Solid Edge part; units mm, degrees
sketch "Sketch1" plane through (0, 0, 0) normal (0, 0, 1) x (1, 0, 0)
  line L0 (-28, -63) -> (28, -63)
  line L1 (28, -63) -> (28, 24)
  line L2 (28, 24) -> (-28, 24)
  line L3 (-28, 24) -> (-28, -63)
  circle A0 centre (-23, -43) radius 1.7
  circle A1 centre (23, -43) radius 1.7
  circle A2 centre (-23, 18) radius 1.7
  circle A3 centre (23, 18) radius 1.7
extrude "Protrusion1" add sketch "Sketch1" along normal blind 6
sketch "Sketch2" plane through (0, 0, 6) normal (0, 0, 1) x (1, 0, 0)
  line L0 (-28, -63) -> (28, -63)
  line L1 (28, -63) -> (28, -55)
  line L2 (28, -55) -> (-28, -55)
  line L3 (-28, -55) -> (-28, -63)
extrude "ExtrudedProtrusion_2" add sketch "Sketch2" along normal blind 24
sketch "Sketch3" plane through (0, 0, 6) normal (0, 0, 1) x (1, 0, 0)
  line L0 (-28, -55) -> (-20, -55)
  line L1 (-20, -55) -> (-28, -20)
  line L2 (-28, -20) -> (-28, -55)
extrude "ExtrudedProtrusion_3" add sketch "Sketch3" along normal blind 20
sketch "Sketch4" plane through (0, 0, 6) normal (0, 0, 1) x (1, 0, 0)
  line L0 (28, -55) -> (20, -55)
  line L1 (20, -55) -> (28, -20)
  line L2 (28, -20) -> (28, -55)
extrude "ExtrudedProtrusion_4" add sketch "Sketch4" along normal blind 20
sketch "Sketch5" plane through (0, -55, 0) normal (0, -1, 0) x (1, 0, 0)
  circle A0 centre (-20, 18.7) radius 1.7
  circle A1 centre (20, 18.7) radius 1.7
extrude "ExtrudedCutout_1" cut sketch "Sketch5" along normal blind 8
Input: part model. Units: mm. Frame: model coordinates. A direction names the side the tool comes from. Round coordinates to 2 decimals unless told otherwise and drop trailing zeros. Loops run counter-clockwise (first coordinate to the right, second up) from the corner with the lowest first, then second, coordinate; pieces in that order, holes last.
1) Pull-direction query (Y, two-part tool) for faces 5 (the cylindrical face through (23.8, -41.5, 3)), 6 (the flat face through (0, -63, 15)), 7 (the flat face through (23.944, -37.745, 15.86)), 8 (the cylindrical face through (-23.37, -41.34, 2.96)); classes: released by +Y, released by -Y, zero draft, split by the parting line, or undercut.
Ans:
face 5: undercut
face 6: released by -Y
face 7: released by +Y
face 8: undercut
2) Section query C-C on z = 8.5. Return the cut outline in (x, y), plus the area to 3 significant figures.
Ans:
outline: (-28, -63) - (28, -63) - (28, -20) - (20, -55) - (-20, -55) - (-28, -20) - close
area: 728 mm2
3) Section query A-A on y = 18. Return the cut outline in (x, z), plus the area to 3 significant figures.
Ans:
outline: (-28, 0) - (-24.7, 0) - (-24.7, 6) - (-28, 6) - close; (-21.3, 0) - (21.3, 0) - (21.3, 6) - (-21.3, 6) - close; (24.7, 0) - (28, 0) - (28, 6) - (24.7, 6) - close
area: 295 mm2
4) Set-up query: faces 1 (the flat face through (-26, -45, 26)), 2 (the flat face through (-23.944, -37.745, 15.86)), 3 (the flat face through (24, -43, 6)), 4 (the cylindrical face through (-18.43, -58.94, 19.35)). Return all of +Z, -Z, +X, -X, +Y, -Y with unobstructed straight access to the full face (end or side cutting, diameter ignored); none if empty.
Ans:
face 1: +Z, +X, -X, +Y
face 2: +Z, +Y
face 3: -Z
face 4: -Y
5) Section query D-D on y = -22. Return the cut outline in (x, z), plus the area to 3 significant figures.
Ans:
outline: (-28, 0) - (28, 0) - (28, 26) - (27.54, 26) - (27.54, 6) - (-27.54, 6) - (-27.54, 26) - (-28, 26) - close
area: 354 mm2
6) Material intervals for line 1 (Y direction, x = -23, z = 3.65); line 2 (X direction, y = -57.25, z = 18.7); line 3 (X direction, y = -43, z = 3.55), sorted ascending.
Ans:
line 1: y = -63 to -44.7, -41.3 to 16.3, 19.7 to 24
line 2: x = -28 to -21.7, -18.3 to 18.3, 21.7 to 28
line 3: x = -28 to -24.7, -21.3 to 21.3, 24.7 to 28
7) Section query B-B on z = 18.7. Return the cut outline in (x, y).
Ans:
outline: (-28, -63) - (-21.7, -63) - (-21.7, -55) - (-20, -55) - (-28, -20) - close; (-18.3, -63) - (18.3, -63) - (18.3, -55) - (-18.3, -55) - close; (20, -55) - (21.7, -55) - (21.7, -63) - (28, -63) - (28, -20) - close
8) Pin query (flat end, axial travel): pin 1 (2.5 mm diameter, centred on x = 23, y = -43, fed in from -Z); pin 2 (5.5 mm diameter, centred on x = -23, y = -43, fed in from +Z); pin 3 (1 mm diameter, centred on x = 2.5, y = 8.5, fed in from +Z). Return the tip coordinate at first contact, or that it passes through.
Ans:
pin 1: stops at z = 6
pin 2: stops at z = 26
pin 3: stops at z = 6
